Source: CAD feature listing. Evaluate the final solid. Frame: model axes, mm. A direction names the side the tool comes from. Round coordinates to 2 decimals unless told otherwise and drop trailing zeros. Loops run counter-clockwise (first coordinate to the right, second up) from the corner with the lowest first, then second, coordinate; pieces in that order, holes last. Notation, with made-up numbers: (-5.75, 84.5) - (43.25, 84.5) arc R25 cw to (43.25, 121.5) - close; hole circle Ø2 at (89.25, 64). An arc over 180 degrees is marked (long way). One line per question, with ' | ' between items. Start each with the question number.
1. Cut plane D-D (z = 3.75). State how many separate pieces and enclosed holes the cut face has, then the cut area to 3 significant figures.
2. Cut plane A-A (x = -45.72). Return loops of the section in (y, z), then the cut area to 3 significant figures.
3. Cut plane C-C (x = -6). Return loops of the section in (y, z), then the cut area to 3 significant figures.
4. Ray query, line 1 (X direction, y = 24.5, z = 4.75); line 2 (Y direction, x = -41, z = 1.25); line 3 (X direction, y = 33.5, z = 4.5). Return the intervals inside material, ascending.
5. Cut plane B-B (y = -15.5). Return loops of the section in (x, z), then the cut area to 3 significant figures.
6. Pin query (flat end, axial travel): pin 1 (4 mm diameter, centred on x = -19.5, z = 3, fed in from -Y); pin 2 (6 mm diameter, centred on x = -12.5, y = -20.5, fed in from -Z); pin 3 (2 mm diameter, centred on x = -13, z = 2, fed in from +Y); pin 4 (4 mm diameter, centred on y = 37, z = 4, fed in from +X). Return the tip coordinate at first contact, or that it passes through.
7. Mould query, pull axis Y, two halves, no side actions, for faces 4 (the flat face through (39, -6.25, 2)), 5 (the flat face through (23, -10, -2)), 6 (the flat face through (-49.223, -39.445, 1.451)). Classes: pulls with the +Y half, pulls with the -Y half, needs draft (parallel to the pull), parting line crosses it, or undercut.
8. Access query for faces 1 (the flat face through (-47, -21.25, 3)), 2 (the flat face through (43.75, -20, 2)), 3 (the flat face through (1, 32.75, 2)). Directions: +Z, -Z, +X, -X, +Y, -Y. A direction counts if a zero-diameter tool reaches every point of the face in a straight line with its end or side. Return the directions, or none.
```python
from build123d import *

# Parameters (mm, degrees)
BOSS_EXTRUDE1_DEPTH   = 5
SHELL1_T              = 6
SKETCH4_W             = 99.5
SKETCH4_H             = 65.5
BOSS_EXTRUDE2_DEPTH   = 2
SKETCH5_W             = 6
SKETCH5_H             = 15.5
CUT_EXTRUDE2_DEPTH    = 5
SKETCH7_R             = 3
SKETCH7_R_2           = 1.75
BOSS_EXTRUDE3_DEPTH   = 7
BOSS_EXTRUDE3_2_DEPTH = 7
BOSS_EXTRUDE3_3_DEPTH = 7
BOSS_EXTRUDE3_4_DEPTH = 7
BOSS_EXTRUDE4_DEPTH   = 7


with BuildPart() as part:
    # Sketch1 → Boss-Extrude1 (new body)
    with BuildSketch(Plane.XY):
        Polygon((43.75, 26.75), (-43.75, 26.75), (-43.75, -26.75), (43.75, -26.75), (43.75, -12.25), (21.75, -12.25), (21.75, 12.25), (43.75, 12.25), align=None)
    extrude(amount=BOSS_EXTRUDE1_DEPTH)

    # Shell1
    shell1_openings = [part.faces().sort_by_distance(p)[0] for p in [
        (-4.261512463, 0, 0),
        (-4.261512463, 0, 5),
    ]]
    offset(amount=SHELL1_T, openings=shell1_openings, kind=Kind.INTERSECTION)

    # Sketch4 → Boss-Extrude2 (add)
    with BuildSketch(Plane(origin=(0, 0, 0), x_dir=(-1, 0, 0), z_dir=(0, 0, -1))):
        Rectangle(SKETCH4_W, SKETCH4_H)
        Polygon((-42.75, 12.25), (-42.75, 25.75), (42.75, 25.75), (42.75, -25.75), (-42.75, -25.75), (-42.75, -12.25), (-21.75, -12.25), (-21.75, 12.25), align=None, mode=Mode.SUBTRACT)
    extrude(amount=BOSS_EXTRUDE2_DEPTH)

    # Sketch5 → Cut-Extrude2 (cut)
    with BuildSketch(Plane.XY.offset(5)):
        with Locations((-46.75, -13.5)):
            Rectangle(SKETCH5_W, SKETCH5_H)
    extrude(amount=-CUT_EXTRUDE2_DEPTH, mode=Mode.SUBTRACT)



with BuildPart() as body_2:
    # Sketch7 → Boss-Extrude3 (new body)
    with BuildSketch(Plane(origin=(0, 0, -2), x_dir=(-1, 0, 0), z_dir=(0, 0, -1))):
        with Locations((-45.72, 45.72)):
            Circle(SKETCH7_R)
        with Locations((-45.72, 45.72)):
            Circle(SKETCH7_R_2, mode=Mode.SUBTRACT)
    extrude(amount=-BOSS_EXTRUDE3_DEPTH)


with BuildPart() as body_3:
    # Sketch7 → Boss-Extrude3 2 (new body)
    with BuildSketch(Plane(origin=(0, 0, -2), x_dir=(-1, 0, 0), z_dir=(0, 0, -1))):
        with Locations((45.72, 45.72)):
            Circle(SKETCH7_R)
        with Locations((45.72, 45.72)):
            Circle(SKETCH7_R_2, mode=Mode.SUBTRACT)
    extrude(amount=-BOSS_EXTRUDE3_2_DEPTH)


with BuildPart() as body_4:
    # Sketch7 → Boss-Extrude3 3 (new body)
    with BuildSketch(Plane(origin=(0, 0, -2), x_dir=(-1, 0, 0), z_dir=(0, 0, -1))):
        with Locations((45.72, -45.72)):
            Circle(SKETCH7_R)
        with Locations((45.72, -45.72)):
            Circle(SKETCH7_R_2, mode=Mode.SUBTRACT)
    extrude(amount=-BOSS_EXTRUDE3_3_DEPTH)


with BuildPart() as body_5:
    # Sketch7 → Boss-Extrude3 4 (new body)
    with BuildSketch(Plane(origin=(0, 0, -2), x_dir=(-1, 0, 0), z_dir=(0, 0, -1))):
        with Locations((-45.72, -45.72)):
            Circle(SKETCH7_R)
        with Locations((-45.72, -45.72)):
            Circle(SKETCH7_R_2, mode=Mode.SUBTRACT)
    extrude(amount=-BOSS_EXTRUDE3_4_DEPTH)


with BuildPart() as part_1:
    add(part.part)

    add(body_2.part)  # Boss-Extrude4 merges body 2

    add(body_3.part)  # Boss-Extrude4 merges body 3

    add(body_4.part)  # Boss-Extrude4 merges body 4

    add(body_5.part)  # Boss-Extrude4 merges body 5
    # Sketch8 → Boss-Extrude4 (add)
    with BuildSketch(Plane(origin=(0, 0, -2), x_dir=(-1, 0, 0), z_dir=(0, 0, -1))):
        with BuildLine():
            Line((-48.71075267, 45.955368794), (-49.75, 32.75))
            Line((-49.75, 32.75), (-41.69, 32.75))
            Line((-41.69, 32.75), (-42.72924733, 45.955368794))
            ThreePointArc((-42.72924733, 45.955368794), (-42.722312724, 45.837775191), (-42.72, 45.72))
            ThreePointArc((-42.72, 45.72), (-45.837775191, 42.722312724), (-48.71075267, 45.955368794))
        make_face()
        with BuildLine():
            Line((42.72924733, 45.955368794), (41.69, 32.75))
            Line((41.69, 32.75), (49.75, 32.75))
            Line((49.75, 32.75), (48.71075267, 45.955368794))
            ThreePointArc((48.71075267, 45.955368794), (48.717687276, 45.837775191), (48.72, 45.72))
            ThreePointArc((48.72, 45.72), (45.602224809, 42.722312724), (42.72924733, 45.955368794))
        make_face()
        with BuildLine():
            Line((49.75, -32.75), (41.69, -32.75))
            Line((41.69, -32.75), (42.72924733, -45.955368794))
            ThreePointArc((42.72924733, -45.955368794), (45.602224809, -42.722312724), (48.72, -45.72))
            ThreePointArc((48.72, -45.72), (48.717687276, -45.837775191), (48.71075267, -45.955368794))
            Line((48.71075267, -45.955368794), (49.75, -32.75))
        make_face()
        with BuildLine():
            Line((-42.72924733, -45.955368794), (-41.69, -32.75))
            Line((-41.69, -32.75), (-49.75, -32.75))
            Line((-49.75, -32.75), (-48.71075267, -45.955368794))
            ThreePointArc((-48.71075267, -45.955368794), (-45.837775191, -42.722312724), (-42.72, -45.72))
            ThreePointArc((-42.72, -45.72), (-42.722312724, -45.837775191), (-42.72924733, -45.955368794))
        make_face()
    extrude(amount=-BOSS_EXTRUDE4_DEPTH)


solid = part_1.part
```
Answers follow:
1) separate pieces: 1 | enclosed holes: 4 | area: 2,390 mm2
2) outline: (-48.72, -2) - (-47.47, -2) - (-47.47, 5) - (-48.72, 5) - close; (-43.97, -2) - (43.97, -2) - (43.97, 5) - (-5.75, 5) - (-5.75, 0) - (-21.25, 0) - (-21.25, 5) - (-43.97, 5) - close; (47.47, -2) - (48.72, -2) - (48.72, 5) - (47.47, 5) - close | area: 556 mm2
3) outline: (-32.75, -2) - (-25.75, -2) - (-25.75, 0) - (-26.75, 0) - (-26.75, 5) - (-32.75, 5) - close; (25.75, -2) - (32.75, -2) - (32.75, 5) - (26.75, 5) - (26.75, 0) - (25.75, 0) - close | area: 88.0 mm2
4) line 1: x = -49.75 to -43.75, 43.75 to 49.75 | line 2: y = -32.75 to -26.75, 26.75 to 32.75 | line 3: x = -49.69 to -41.75, 41.75 to 49.69
5) outline: (-49.75, -2) - (-42.75, -2) - (-42.75, 0) - (-49.75, 0) - close; (42.75, -2) - (49.75, -2) - (49.75, 5) - (43.75, 5) - (43.75, 0) - (42.75, 0) - close | area: 58.0 mm2
6) pin 1: stops at y = -32.75 | pin 2: passes through | pin 3: stops at y = 32.75 | pin 4: stops at x = 49.57
7) face 4: undercut | face 5: needs draft | face 6: pulls with the -Y half
8) face 1: +Z, -X | face 2: +Z | face 3: +Z, -Z, +Y
